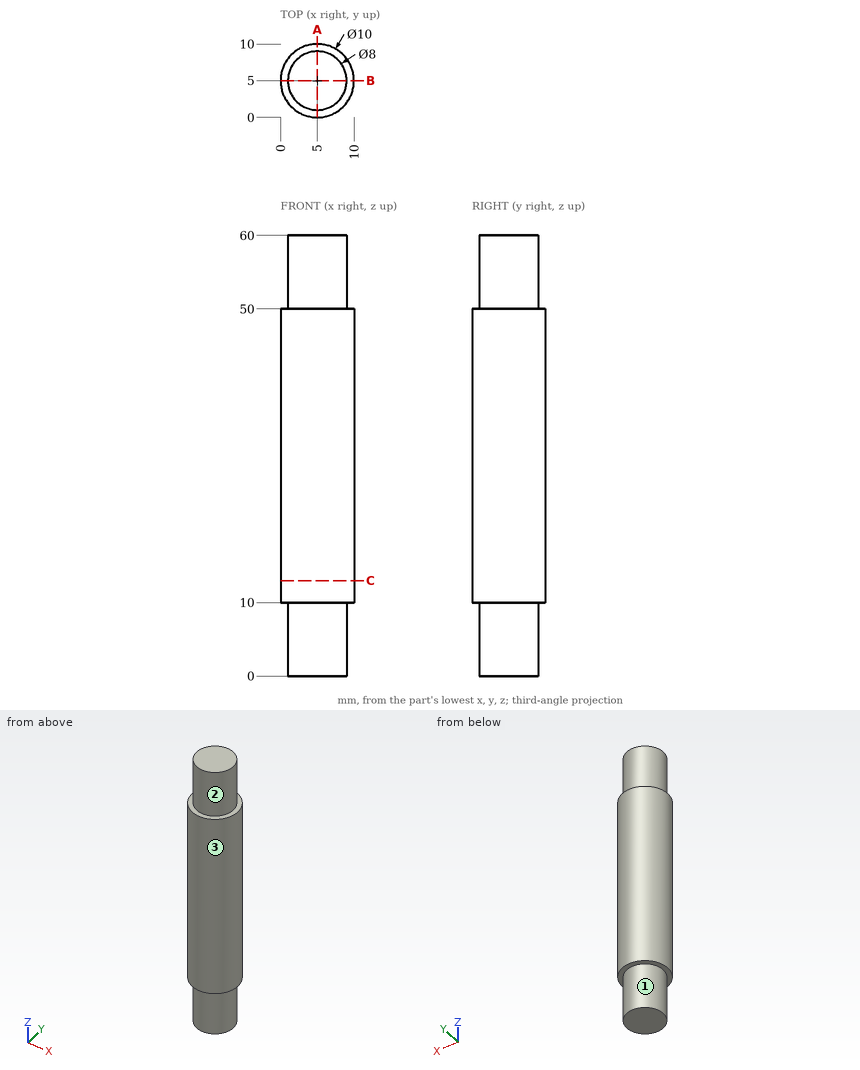
Print and shaded views of the part. All mm, measured from the part's lowest x, y and z. A direction names the side the tool comes from. Give positions to 0.01 mm unless a question says otherwise; leave off trailing zeros. Write each loop counter-clockwise with the first axis right and the second up, starting at its lowest first coordinate (ties: lowest second). Pieces come first, ordered by that corner, then holes. Notation, with made-up numbers: (58.5, 81.25) -> (93.5, 81.25) arc R23 cw to (93.5, 120.25) -> close; hole circle Ø1 at (47, -11.5). An arc over 180 degrees is marked (long way). Use CSV: the item, a comma, the result in double quotes. Start each with the question number.
1) Pin check, flat tips, straight feed: P1, Ø1, axis at x = 6.5, z = 37.5, coming from the -Y side; P2, Ø2, axis at y = 7.5, z = 31.5, coming from the +X side; P3, Ø2, axis at y = 8.5, z = 18.5, coming from the +X side; P4, Ø4, axis at y = 7, z = 23, coming from the +X side. Stop position of each tip, or through.
2) Drill centre lines: L1, parallel to Z at x = 9.75, y = 5.5; L2, parallel to X at y = 8, z = 21; L3, parallel to X at y = 4.75, z = 23.5. Where is each one in solid material? Low to high.
3) Cut at A-A on x = 5. List the corners of the cut face in (y, z).
4) Tool access for the marked faces 1, 2 and 3: list every direction of +Z, -Z, +X, -X, +Y, -Y with a clear straight run to the whole face (end or side of a thin tool).
5) Cut at C-C on z = 13. List the corners of the cut face in (x, y).
Final values:
1,P1,"stops at y = 0.1"
1,P2,"stops at x = 9.77"
1,P3,"stops at x = 9.33"
1,P4,"stops at x = 10"
2,L1,"z = 10 to 50"
2,L2,"x = 1 to 9"
2,L3,"x = 0.01 to 9.99"
3,outline,"(0, 10) -> (1, 10) -> (1, 0) -> (9, 0) -> (9, 10) -> (10, 10) -> (10, 50) -> (9, 50) -> (9, 60) -> (1, 60) -> (1, 50) -> (0, 50) -> close"
4,face 1,"-Z"
4,face 2,"+Z"
4,face 3,"+Z, -Z"
5,outline,"circle Ø10 at (5, 5)"
